Source: three-view drawing plus pictorial views. Frame: mm from the lowest corner of the part. A direction names the side the tool comes from. Give positions to 0.01 mm unless a question says otherwise; leave off trailing zeros. Order: outer loops, then holes, each group sorted by start corner. A loop starts at its lowest first (then second) coordinate and runs counter-clockwise, first axis right, second up. Notation, with made-up numbers: M 73,23.5 L 109,23.5 A23 cw 109,48.5 Z; hole C 16,-38.5 d3. An arc over 180 degrees is marked long. Use CSV: the item, a comma, the result in double quotes.
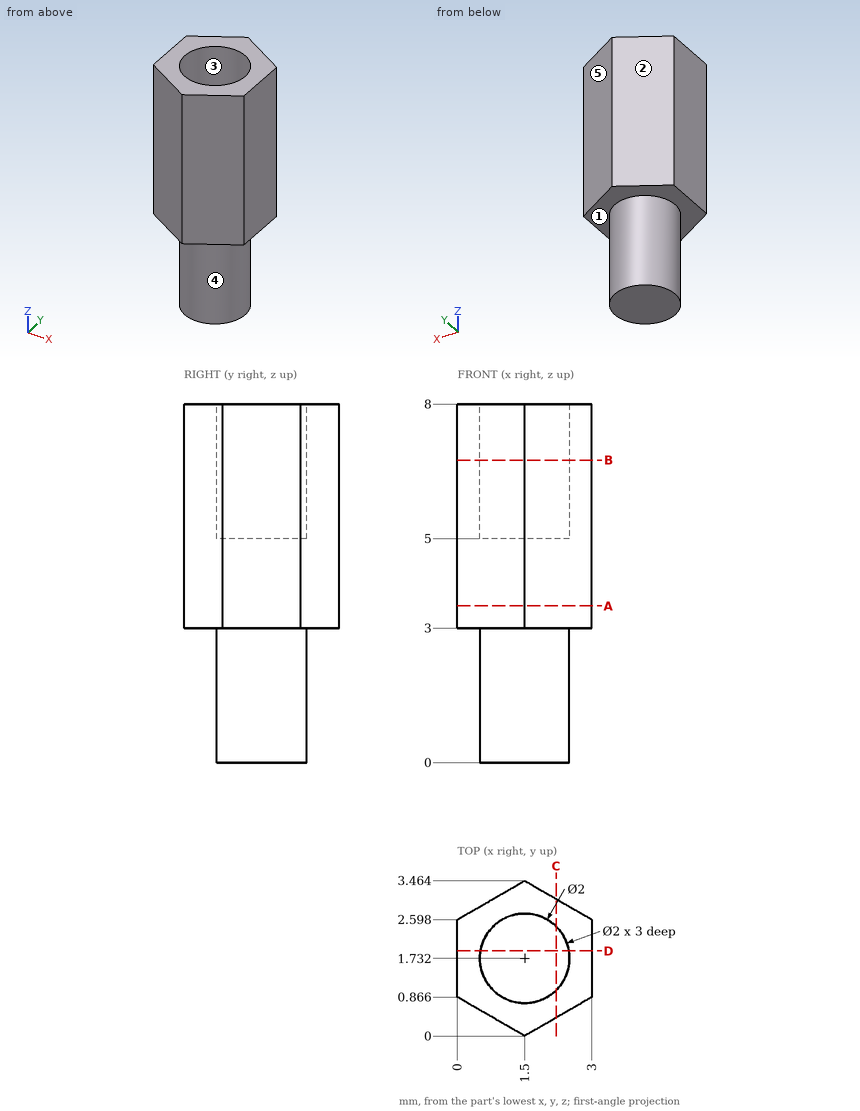
1. Pull-direction query (Y, two-part tool) for the marked faces 3, 4 and 5; classes: +Y half, -Y half, draft (parallel to the pull), parting line (faces both ways), or undercut.
Answer:
face 3,"undercut"
face 4,"parting line"
face 5,"+Y half"
2. Line query: line 1 (Z direction, x = 0.9, y = 0.85); line 2 (Z direction, x = 1.45, y = 1.6); line 3 (X direction, y = 2.5, z = 0.5). Output: solid intervals per line, ascending.
Answer:
line 1,"3 to 8"
line 2,"0 to 5"
line 3,"0.86 to 2.14"
3. Section B-B, the plane z = 6.75. Return the cut outline in (x, y).
Answer:
outline,"M 0,0.87 L 1.5,0 L 3,0.87 L 3,2.6 L 1.5,3.46 L 0,2.6 Z; hole C 1.5,1.73 d2"
4. Section D-D, the plane y = 1.9. Return the cut outline in (x, z).
Answer:
outline,"M 0,3 L 0.51,3 L 0.51,0 L 2.49,0 L 2.49,3 L 3,3 L 3,8 L 2.49,8 L 2.49,5 L 0.51,5 L 0.51,8 L 0,8 Z"
5. Pin query (flat end, axial travel): pin 1 Ø1.5 at (x, z) = (1, 5) entering from -Y; pin 2 Ø1.5 at (x, z) = (0.5, 2) entering from +Y; pin 3 Ø1.2 at (x, y) = (1.5, 1.73) entering from +Z. Return the tip coordinate at first contact, or that it passes through.
Answer:
pin 1,"y = 0"
pin 2,"y = 2.7"
pin 3,"z = 5"
6. Section C-C, the plane x = 2.2. Return the cut outline in (y, z).
Answer:
outline,"M 0.4,3 L 1.02,3 L 1.02,0 L 2.45,0 L 2.45,3 L 3.06,3 L 3.06,8 L 2.45,8 L 2.45,5 L 1.02,5 L 1.02,8 L 0.4,8 Z"
7. Section A-A, the plane z = 3.5. Return the cut outline in (x, y).
Answer:
outline,"M 0,0.87 L 1.5,0 L 3,0.87 L 3,2.6 L 1.5,3.46 L 0,2.6 Z"
8. Reachability of the marked faces 1 and 2 from +Z, -Z, +X, -X, +Y, -Y: full face, straight path, thin tool, end or side. Return the list, or none.
Answer:
face 1,"-Z"
face 2,"+Z, -Z, -X, +Y"
